Design review of the part built by this model. Coordinates are the model's own, in mm. A direction names the side the tool comes from. Round coordinates to 2 decimals unless told otherwise and drop trailing zeros. Order: outer loops, then holes, each group sorted by start corner. A loop starts at its lowest first (then second) coordinate and runs counter-clockwise, first axis right, second up. Notation, with made-up numbers: M 69,48 L 94,48 A27 cw 94,65 Z; hole C -10.5,0 d6. An arc over 180 degrees is marked long. Use a Markdown table: item, result. Add a question column.
(1) To check wall thickness, follow probe 1 along Y at (x, z) = (8, 16.75); probe 2 along Z at (x, y) = (-7, -0.5); probe 3 along X at (y, z) = (2, 10.25). State the ranges of each line that lie inside material, in increasing order. Write a range as from..to.
(2) The part is to be moulded in two halves that separate along Y. For faces 1 (the face through (0, 5, 15)), 2 (the face through (-25, 0, 10)), 3 (the face through (5, -25, 10)), 4 (the face through (-15, 0, 15)), say which applies: released by +Y, released by -Y, zero draft, split by the parting line, or undercut.
(3) For pin 1 (2 mm diameter, centred on x = 4, y = 17, fed in from -Z); pin 2 (2 mm diameter, centred on y = 19, z = 13.5, fed in from +X); pin 3 (4 mm diameter, centred on x = 16.5, z = 8, fed in from +Y), all flat-tipped, find the tip position at first contact; note any pin that passes through.
(4) Take a section at B-B (y = 0). Write out the cut boundary in (x, z), then the cut area to 3 significant figures.
(5) Machinability: for faces 5 (the face through (15, 0, 15)), 6 (the face through (-0.3, -5.2, 20)), which of the approach directions +Z, -Z, +X, -X, +Y, -Y give a long, thin tool a straight path to every point of the face, cutting with its end or side? Answer none if there is none.
(6) Take a section at C-C (x = 9). Write out the cut boundary in (y, z).
(7) Take a section at A-A (z = 17.5). Write out the cut boundary in (x, y).
```python
from build123d import *

# Parameters (mm, degrees)
SKETCH_W     = 50
SKETCH_H     = 50
PAD_DEPTH    = 20
POCKET_DEPTH = 10
FILLET_R     = 11


with BuildPart() as part:
    # Sketch → Pad (new body)
    with BuildSketch(Plane.XY):
        Rectangle(SKETCH_W, SKETCH_H)
    extrude(amount=PAD_DEPTH)

    # Sketch001 → Pocket (cut)
    with BuildSketch(Plane.XY.offset(20)):
        with BuildLine():
            ThreePointArc((-10, 5), (-15, 0), (-10, -5))
            Line((-10, -5), (10, -5))
            ThreePointArc((10, -5), (15, 0), (10, 5))
            Line((-10, 5), (10, 5))
        make_face()
    extrude(amount=-POCKET_DEPTH, mode=Mode.SUBTRACT)

    # Fillet
    fillet_edges = [part.edges().sort_by_distance(p)[0] for p in [
        (-25, -25, 10),
        (-25, 25, 10),
        (25, 25, 10),
    ]]
    fillet(fillet_edges, radius=FILLET_R)


solid = part.part
```
Verdict:
| question | item | result |
|---|---|---|
| 1 | probe 1 | y = -25..-5, 5..25 |
| 1 | probe 2 | z = 0..10 |
| 1 | probe 3 | x = -25..-14.58, 14.58..25 |
| 2 | face 1 | undercut |
| 2 | face 2 | zero draft |
| 2 | face 3 | released by -Y |
| 2 | face 4 | undercut |
| 3 | pin 1 | stops at z = 0 |
| 3 | pin 2 | stops at x = 24.25 |
| 3 | pin 3 | stops at y = 24.99 |
| 4 | outline | M -25,0 L 25,0 L 25,20 L 15,20 L 15,10 L -15,10 L -15,20 L -25,20 Z |
| 4 | area | 700 mm^2 |
| 5 | face 5 | +Z |
| 5 | face 6 | +Z, +X, -X, +Y, -Y |
| 6 | outline | M -25,0 L 25,0 L 25,20 L 5,20 L 5,10 L -5,10 L -5,20 L -25,20 Z |
| 7 | outline | M -25,-14 A11 ccw -14,-25 L 25,-25 L 25,14 A11 ccw 14,25 L -14,25 A11 ccw -25,14 Z; hole M -10,-5 L 10,-5 A5 ccw 10,5 L -10,5 A5 ccw Z |
